Autodesk Inventor part; units mm, degrees
ref_plane "YZ Plane" through (0, 0, 0) normal (1, 0, 0) x (0, 1, 0)
ref_plane "XZ Plane" through (0, 0, 0) normal (0, 1, 0) x (-1, 0, 0)
ref_plane "XY Plane" through (0, 0, 0) normal (0, 0, 1) x (1, 0, 0)
sketch "스케치1" plane through (0, 0, 0) normal (0, 0, 1) x (1, 0, 0)
  circle A0 centre (-7.7782, -7.7782) radius 1.55
  circle A1 centre (7.7782, -7.7782) radius 1.55
  circle A2 centre (7.7782, 7.7782) radius 1.55
  circle A3 centre (-7.7782, 7.7782) radius 1.55
  circle A4 centre (0, 11) radius 1.55
  circle A5 centre (11, 0) radius 1.55
  circle A6 centre (0, -11) radius 1.55
  circle A7 centre (-11, 0) radius 1.55
  circle A8 centre (0, 0) radius 14
  arc A9 (0, -5.2) -> (0, 5.2) centre (0, 0) ccw
  line L0 (32.5, -23) -> (32.5001, 127)
  line L1 (26.5, -23) -> (32.5, -23)
  line L2 (26.5001, 127) -> (26.5, -23)
  line L3 (32.5001, 127) -> (26.5001, 127)
  line L4 (0, 14) -> (32.5, 14)
  line L5 (32.5, 14) -> (32.5, -12.55)
  line L6 (0, -12.55) -> (0, 14)
  line L7 (0, -14) -> (32.5, -14)
  line L8 (32.5, -14) -> (32.5, -12.55)
  line L9 (0, 5.2) -> (-9.6, 5.2)
  line L10 (-9.6, -5.2) -> (0, -5.2)
  line L11 (0, -5.2) -> (0, 5.2)
  arc A10 (-11.2, -8.4) -> (-11.2, 8.4) centre (0, 0) ccw
  arc A11 (-11.2, 8.4) -> (-9.6, 5.2) centre (-9.6, 7.2) ccw
  arc A12 (-9.6, -5.2) -> (-11.2, -8.4) centre (-9.6, -7.2) ccw
  line L12 (26.5, 0) -> (32.5, 0)
  line L13 (32.5, 0) -> (32.5, -3)
  line L14 (32.5, -3) -> (26.5, -3)
  line L15 (26.5, -3) -> (26.5, 0)
  line L16 (32.5, 0) -> (26.5, 0)
  line L17 (26.5, 0) -> (26.5, 3)
  line L18 (26.5, 3) -> (32.5, 3)
  line L19 (32.5, 3) -> (32.5, 0)
  point P0 (0, 0)
  point P1 (-12.9985, -5.2)
  point P2 (-12.9985, 5.2)
  point P3 (-11.2, 8.4)
  dimension "d1" = 2
  dimension "d4" = 3
  dimension "d5" = 3
extrude "돌출1" add sketch "스케치1" along normal blind 6 contours A4 L6 A8 A12 L10 A9 | A4 L6 L9 A11 A8 | L4 L2 L7 A8 | L4 L0 L18 L2 | L18 L0 L12 L2 | L2 L14 L0 L7 | L12 L0 L14 L2
sketch "스케치2" plane through (0, 0, 6) normal (0, 0, 1) x (1, 0, 0)
  arc A0 (-9.6, -5.2) -> (-11.2, -8.4) centre (-9.6, -7.2) ccw
  arc A1 (-11.2, -8.4) -> (0, -14) centre (0, 0) ccw
  line L0 (0, -14) -> (32.5, -14)
  line L1 (32.5, -14) -> (32.5, 14)
  line L2 (32.5, 14) -> (0, 14)
  arc A2 (0, 14) -> (-11.2, 8.4) centre (0, 0) ccw
  arc A3 (-11.2, 8.4) -> (-9.6, 5.2) centre (-9.6, 7.2) ccw
  line L3 (-9.6, 5.2) -> (0, 5.2)
  arc A4 (0, -5.2) -> (0, 5.2) centre (0, 0) ccw
  line L4 (0, -5.2) -> (-9.6, -5.2)
  circle A5 centre (0, -11) radius 1.55
  circle A6 centre (-7.7782, 7.7782) radius 1.55
  circle A7 centre (-7.7782, -7.7782) radius 1.55
  circle A8 centre (7.7782, -7.7782) radius 1.55
  circle A9 centre (7.7782, 7.7782) radius 1.55
  circle A10 centre (11, 0) radius 1.55
  circle A11 centre (0, 11) radius 1.55
  line L5 (32.5, 14) -> (26.5, 14)
  line L6 (26.5, 14) -> (26.5, -14)
  line L7 (26.5, -14) -> (32.5, -14)
  line L8 (32.5, -14) -> (32.5, 14)
  line L9 (32.5, -14) -> (32.5, 14)
  line L10 (32.5, 0) -> (26.5, 0)
  line L11 (26.5, 0) -> (26.5, -3)
  line L12 (26.5, -3) -> (32.5, -3)
  line L13 (32.5, -3) -> (32.5, 0)
  line L14 (32.5, 0) -> (26.5, 0)
  line L15 (26.5, 0) -> (26.5, 3)
  line L16 (26.5, 3) -> (32.5, 3)
  line L17 (32.5, 3) -> (32.5, 0)
  point P0 (0, 0)
  point P1 (32.5, -3)
  dimension "d6" = 6
  dimension "d7" = 3
  dimension "d8" = 3
extrude "돌출2" cut sketch "스케치2" against normal blind 6 contours L6 L12 L1 L0 | L6 L2 L1 L16
sketch "스케치3" plane through (32.5, 52, -3.7) normal (1, 0, 0) x (0, -1, 0)
  point P0 (52, -3.7)
sketch "스케치4" plane through (26.5, -14, 6) normal (1, 0, 0) x (0, 0, -1)
  circle A0 centre (3, 5.5) radius 1.35
  circle A1 centre (3, 22.5) radius 1.35
  circle A2 centre (66.3, 80.5) radius 1.3
  circle A3 centre (66.3, 51.5) radius 1.3
  circle A4 centre (66.3, 118) radius 1.35
  circle A5 centre (66.3, 14) radius 1.35
  arc A6 (62.1, 141) -> (63.1, 140) centre (63.1, 141) ccw
  line L0 (62.1, 141) -> (-10.1, 141)
  line L1 (-10.1, 141) -> (-10.1, -9)
  line L2 (-10.1, -9) -> (62.1, -9)
  arc A7 (63.1, -8) -> (62.1, -9) centre (63.1, -9) ccw
  line L3 (63.1, -8) -> (63.1, -3.8)
  arc A8 (64.1, -2.8) -> (63.1, -3.8) centre (63.1, -2.8) ccw
  line L4 (64.1, -2.8) -> (68.3, -2.8)
  arc A9 (69.3, -1.8) -> (68.3, -2.8) centre (69.3, -2.8) ccw
  line L5 (69.3, -1.8) -> (69.3, 29.8)
  arc A10 (68.3, 30.8) -> (69.3, 29.8) centre (69.3, 30.8) ccw
  line L6 (68.3, 30.8) -> (64.1, 30.8)
  arc A11 (63.1, 31.8) -> (64.1, 30.8) centre (63.1, 30.8) ccw
  line L7 (63.1, 31.8) -> (63.1, 36.2)
  arc A12 (64.1, 37.2) -> (63.1, 36.2) centre (63.1, 37.2) ccw
  line L8 (64.1, 37.2) -> (68.3, 37.2)
  arc A13 (69.3, 38.2) -> (68.3, 37.2) centre (69.3, 37.2) ccw
  line L9 (69.3, 38.2) -> (69.3, 93.8)
  arc A14 (68.3, 94.8) -> (69.3, 93.8) centre (69.3, 94.8) ccw
  line L10 (68.3, 94.8) -> (64.1, 94.8)
  arc A15 (63.1, 95.8) -> (64.1, 94.8) centre (63.1, 94.8) ccw
  line L11 (63.1, 95.8) -> (63.1, 100.2)
  arc A16 (64.1, 101.2) -> (63.1, 100.2) centre (63.1, 101.2) ccw
  line L12 (64.1, 101.2) -> (68.3, 101.2)
  arc A17 (69.3, 102.2) -> (68.3, 101.2) centre (69.3, 101.2) ccw
  line L13 (69.3, 102.2) -> (69.3, 133.8)
  arc A18 (68.3, 134.8) -> (69.3, 133.8) centre (69.3, 134.8) ccw
  line L14 (68.3, 134.8) -> (64.1, 134.8)
  arc A19 (63.1, 135.8) -> (64.1, 134.8) centre (63.1, 134.8) ccw
  line L15 (63.1, 135.8) -> (63.1, 140)
  arc A20 (0.8, 121.2) -> (-0.2, 120.2) centre (-0.2, 121.2) ccw
  line L16 (0.8, 121.2) -> (5.2, 121.2)
  arc A21 (6.2, 120.2) -> (5.2, 121.2) centre (6.2, 121.2) ccw
  line L17 (6.2, 120.2) -> (6.2, 115.8)
  arc A22 (5.2, 114.8) -> (6.2, 115.8) centre (6.2, 114.8) ccw
  line L18 (5.2, 114.8) -> (0.8, 114.8)
  arc A23 (-0.2, 115.8) -> (0.8, 114.8) centre (-0.2, 114.8) ccw
  line L19 (-0.2, 115.8) -> (-0.2, 120.2)
  arc A24 (0.8, 17.2) -> (-0.2, 16.2) centre (-0.2, 17.2) ccw
  line L20 (0.8, 17.2) -> (5.2, 17.2)
  arc A25 (6.2, 16.2) -> (5.2, 17.2) centre (6.2, 17.2) ccw
  line L21 (6.2, 16.2) -> (6.2, 11.8)
  arc A26 (5.2, 10.8) -> (6.2, 11.8) centre (6.2, 10.8) ccw
  line L22 (5.2, 10.8) -> (0.8, 10.8)
  arc A27 (-0.2, 11.8) -> (0.8, 10.8) centre (-0.2, 10.8) ccw
  line L23 (-0.2, 11.8) -> (-0.2, 16.2)
  circle A28 centre (29.5, 66) radius 1.6
  point P0 (6, 14)
extrude "돌출3" cut sketch "스케치4" against normal blind 6 contours A0 | A1
properties part number "부품69" material "PMMA 플라스틱"
Geometry: final body of the model. Coordinates: model frame, mm. A direction names the side the tool comes from. Round coordinates to 2 decimals unless told otherwise and drop trailing zeros. Order: outer loops, then holes, each group sorted by start corner. A loop starts at its lowest first (then second) coordinate and runs counter-clockwise, first axis right, second up. Notation, with made-up numbers: (27.5, -28.75) -> (34.5, -28.75) arc R25 ccw to (34.5, 6.25) -> close; hole circle Ø10 at (17, -32). An arc over 180 degrees is marked (long way). Use one line per item in the form item = value. Start each with the question number.
1. Cut plane A-A (x = 11). Return the cut outline in (y, z).
2. Draft query along Y for faces 4 (the face through (29, 3, 3)), 5 (the face through (29, -3, 3)), 6 (the face through (26.5, -7, 4)), 7 (the face through (20.5, -8, 3)). Return one class per face: pulls with the +Y half, pulls with the -Y half, needs draft (parallel to the pull), parting line crosses it, or undercut.
3. Reachability of faces 1 (the face through (23.542, 9.839, 3.176)), 2 (the face through (26.5, 10, 4)), 3 (the face through (-5, 5.2, 3)) from +Z, -Z, +X, -X, +Y, -Y: full face, straight path, thin tool, end or side. Return the list, or none.
4. Cut plane D-D (x = 1). Return the cut outline in (y, z), then the cut area to 3 significant figures.
5. Cut plane C-C (z = 0.5). Return the cut outline in (x, y), then the cut area to 3 significant figures.
6. Pin query (flat end, axial travel): pin 1 Ø2.5 at (x, y) = (11, 0) entering from +Z; pin 2 Ø3.5 at (x, y) = (-7.78, -7.78) entering from -Z; pin 3 Ø3.5 at (y, z) = (-8.5, 3) entering from +X; pin 4 Ø3 at (x, z) = (-3, 3.5) entering from +Y. Return the tip coordinate at first contact, or that it passes through.
7. Cut plane B-B (y = 0). Return the cut outline in (x, z), then the cut area to 3 significant figures.
8. Line query: probe 1 along Y at (x, z) = (0, 4.35); probe 2 along Y at (x, z) = (-8, 5.7); probe 3 along X at (y, z) = (6.75, 4.45). Output: solid intervals per line, ascending.
Solution:
q1.outline = (-14, 0) -> (-1.55, 0) -> (-1.55, 6) -> (-14, 6) -> close; (1.55, 0) -> (14, 0) -> (14, 6) -> (1.55, 6) -> close
q2.face_4 = pulls with the +Y half
q2.face_5 = pulls with the -Y half
q2.face_6 = needs draft
q2.face_7 = undercut
q3.face_1 = +X
q3.face_2 = +Z, -Z, +X, +Y
q3.face_3 = +Z, -Z, -X
q4.outline = (-14, 0) -> (-12.18, 0) -> (-12.18, 6) -> (-14, 6) -> close; (-9.82, 0) -> (-5.1, 0) -> (-5.1, 6) -> (-9.82, 6) -> close; (5.1, 0) -> (9.82, 0) -> (9.82, 6) -> (5.1, 6) -> close; (12.18, 0) -> (14, 0) -> (14, 6) -> (12.18, 6) -> close
q4.area = 78.3 mm^2
q5.outline = (-11.2, -8.4) arc R14 ccw to (0, -14) -> (26.5, -14) -> (26.5, -3) -> (32.5, -3) -> (32.5, 3) -> (26.5, 3) -> (26.5, 14) -> (0, 14) arc R14 ccw to (-11.2, 8.4) arc R2 ccw to (-9.6, 5.2) -> (0, 5.2) arc R5.2 cw to (0, -5.2) -> (-9.6, -5.2) arc R2 ccw to start; hole circle Ø3.1 at (-7.78, -7.78); hole circle Ø3.1 at (-7.78, 7.78); hole circle Ø3.1 at (0, -11); hole circle Ø3.1 at (0, 11); hole circle Ø3.1 at (7.78, -7.78); hole circle Ø3.1 at (7.78, 7.78); hole circle Ø3.1 at (11, 0)
q5.area = 843 mm^2
q6.pin_1 = through
q6.pin_2 = 0
q6.pin_3 = 26.5
q6.pin_4 = 13.92
q7.outline = (5.2, 0) -> (9.45, 0) -> (9.45, 6) -> (5.2, 6) -> close; (12.55, 0) -> (32.5, 0) -> (32.5, 6) -> (12.55, 6) -> close
q7.area = 145 mm^2
q8.probe_1 = -14 to -12.55, -9.45 to -5.2, 5.2 to 9.45, 12.55 to 14
q8.probe_2 = -11.49 to -9.31, -6.24 to -5.2, 5.2 to 6.24, 9.31 to 11.49
q8.probe_3 = -11.55 to -8.94, -6.62 to 6.62, 8.94 to 26.5
